Part print with two shaded views. Sizes in mm from the minimum x, y, z corner. A direction names the side the tool comes from. Coordinates: 2 decimals unless noted, no trailing zeros. Write each loop counter-clockwise with the first axis right and the second up, starting at its lowest first coordinate (ties: lowest second). Pieces come first, ordered by that corner, then holes. Notation, with made-up numbers: (33, 46) - (38, 46) arc R23 ccw to (38, 60) - close; hole circle Ø3 at (15.25, 14.25). An arc over 180 degrees is marked (long way). One line per question, with ' | ' between items. Start each with the question number.
1. Band-saw the part on B-B, the plane x = 3. Write the cut outline in (y, z), then the cut area to 3 significant figures.
2. Band-saw the part on A-A, the plane y = 5. Write the cut outline in (x, z).
3. Band-saw the part on C-C, the plane y = 7.75. Write the cut outline in (x, z).
4. Probe line 1 (Y direction, x = 22, z = 1.4); line 2 (Z direction, x = 7, y = 9); line 3 (Z direction, x = 19.5, y = 7.5). List the from-to ranges inside material, lowest first.
5. Band-saw the part on D-D, the plane x = 12.75. Write the cut outline in (y, z).
6. Flat gauge pins, fed straight in: P1, Ø5, axis at x = 3.5, y = 8.5, coming from the -Z side; P2, Ø4.5, axis at x = 23, y = 3.5, coming from the +Z side; P3, Ø2, axis at x = 15.5, y = 7.5, coming from the -Z side. Where does each tip first touch, or does it go through?
7. Which spindle directions (+Z, -Z, +X, -X, +Y, -Y) get a long thin tool onto all of the face, cutting with end or side? Do the marked faces 1, 2 and 3. Say none if no direction does.
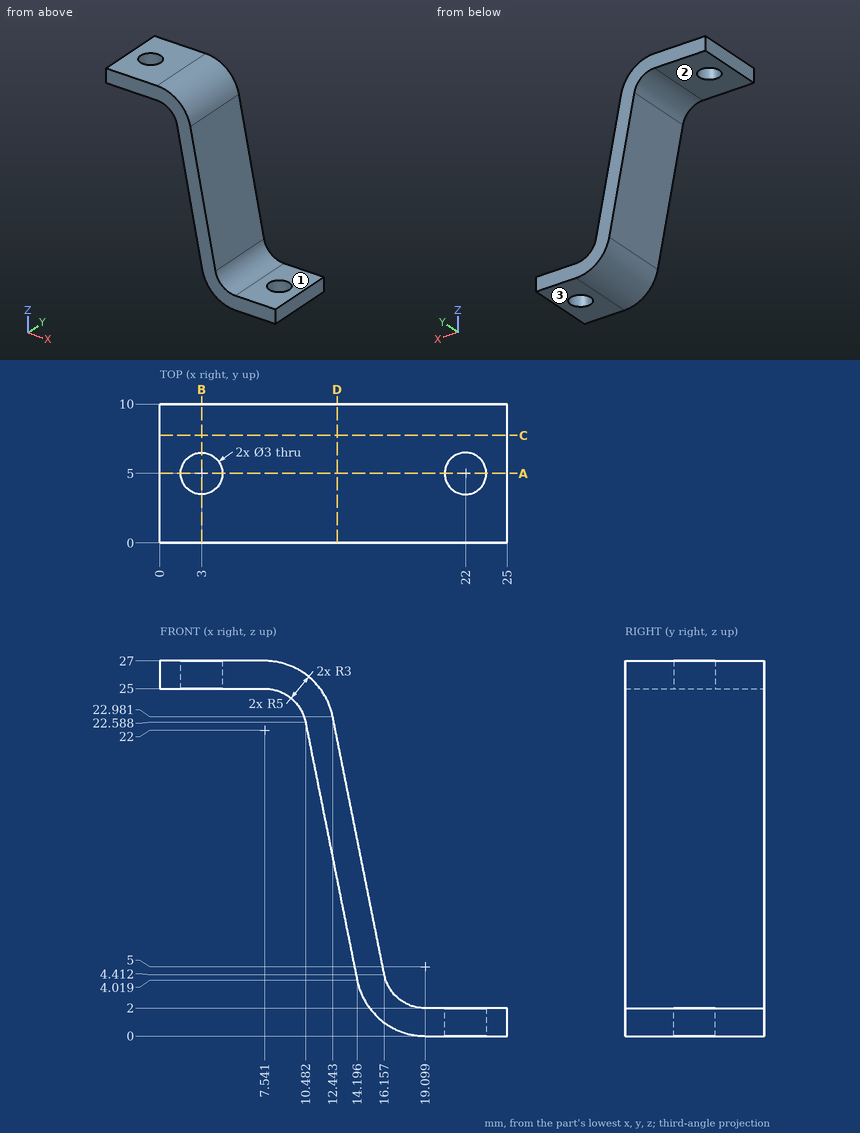
Filled in:
1) outline: (0, 25) - (3.5, 25) - (3.5, 27) - (0, 27) - close; (6.5, 25) - (10, 25) - (10, 27) - (6.5, 27) - close | area: 14.0 mm²
2) outline: (0, 25) - (1.5, 25) - (1.5, 27) - (0, 27) - close; (4.5, 25) - (7.54, 25) arc R3 cw to (10.48, 22.59) - (14.2, 4.02) arc R5 ccw to (19.1, 0) - (20.5, 0) - (20.5, 2) - (19.1, 2) arc R3 cw to (16.16, 4.41) - (12.44, 22.98) arc R5 ccw to (7.54, 27) - (4.5, 27) - close; (23.5, 0) - (25, 0) - (25, 2) - (23.5, 2) - close
3) outline: (0, 25) - (7.54, 25) arc R3 cw to (10.48, 22.59) - (14.2, 4.02) arc R5 ccw to (19.1, 0) - (25, 0) - (25, 2) - (19.1, 2) arc R3 cw to (16.16, 4.41) - (12.44, 22.98) arc R5 ccw to (7.54, 27) - (0, 27) - close
4) line 1: y = 0 to 3.5, 6.5 to 10 | line 2: z = 25 to 27 | line 3: z = 0 to 2
5) outline: (0, 11.25) - (10, 11.25) - (10, 21.45) - (0, 21.45) - close
6) P1: stops at z = 25 | P2: stops at z = 2 | P3: stops at z = 0.73
7) face 1: +Z, +X, +Y, -Y | face 2: -Z, -X, +Y, -Y | face 3: -Z, +X, -X, +Y, -Y
